Geometry check sheet. Reference: the model listing, model coordinates, mm. Face numbers are marked on the shaded views. A direction names the side the tool comes from. Coordinates: 2 decimals unless noted, no trailing zeros. Write each loop counter-clockwise with the first axis right and the second up, starting at its lowest first coordinate (ties: lowest second). Pieces come first, ordered by that corner, then holes. Notation, with made-up numbers: (73.25, 35.5) -> (110.25, 35.5) arc R28 cw to (110.25, 54.5) -> close; hole circle Ø3 at (-40, 82.25). An arc over 180 degrees is marked (long way). Put each result on its own line as item: value. Start each with the question number.
from build123d import *

# Parameters (mm, degrees)
SKETCH1_W           = 25
SKETCH1_H           = 52
BOSS_EXTRUDE1_DEPTH = 2
SKETCH2_W           = 25
SKETCH2_H           = 25
BOSS_EXTRUDE2_DEPTH = 2
SKETCH3_W           = 25
SKETCH3_H           = 25
BOSS_EXTRUDE3_DEPTH = 2
SKETCH5_R           = 4
CUT_EXTRUDE2_DEPTH  = 21
SKETCH6_R           = 1.5
CUT_EXTRUDE3_DEPTH  = 21
SKETCH7_R           = 2.5
CUT_EXTRUDE4_DEPTH  = 81


with BuildPart() as part:
    # Sketch1 → Boss-Extrude1 (new body)
    with BuildSketch(Plane.XY):
        with Locations((-0.174770451, 4.502942624)):
            Rectangle(SKETCH1_W, SKETCH1_H)
    extrude(amount=BOSS_EXTRUDE1_DEPTH)

    # Sketch2 → Boss-Extrude2 (add)
    with BuildSketch(Plane(origin=(0, 30.502942624, 0), x_dir=(1, 0, 0), z_dir=(0, 1, 0))):
        with Locations((-0.174770451, -12.5)):
            Rectangle(SKETCH2_W, SKETCH2_H)
    extrude(amount=BOSS_EXTRUDE2_DEPTH)

    # Sketch3 → Boss-Extrude3 (add)
    with BuildSketch(Plane(origin=(0, -21.497057376, 0), x_dir=(-1, 0, 0), z_dir=(0, -1, 0))):
        with Locations((0.174770451, -12.5)):
            Rectangle(SKETCH3_W, SKETCH3_H)
    extrude(amount=BOSS_EXTRUDE3_DEPTH)

    # Sketch5 → Cut-Extrude2 (cut)
    with BuildSketch(Plane(origin=(0, 0, 0), x_dir=(-1, 0, 0), z_dir=(0, 0, -1))):
        with Locations((0.174770451, 4.502942624)):
            Circle(SKETCH5_R)
    extrude(amount=-CUT_EXTRUDE2_DEPTH, mode=Mode.SUBTRACT)

    # Sketch6 → Cut-Extrude3 (cut)
    with BuildSketch(Plane(origin=(0, 0, 0), x_dir=(-1, 0, 0), z_dir=(0, 0, -1))):
        with Locations((7.174770451, 4.502942624)):
            Circle(SKETCH6_R)
        with Locations((0.174770451, -2.497057376)):
            Circle(SKETCH6_R)
        with Locations((-6.825229549, 4.502942624)):
            Circle(SKETCH6_R)
        with Locations((0.174770451, 11.502942624)):
            Circle(SKETCH6_R)
    extrude(amount=-CUT_EXTRUDE3_DEPTH, mode=Mode.SUBTRACT)

    # Sketch7 → Cut-Extrude4 (cut)
    with BuildSketch(Plane(origin=(0, -23.497057376, 0), x_dir=(-1, 0, 0), z_dir=(0, -1, 0))):
        with Locations(Location((0.174770451, -20, 0), (0, 0, 90))):
            Circle(SKETCH7_R)
    extrude(amount=-CUT_EXTRUDE4_DEPTH, mode=Mode.SUBTRACT)


solid = part.part
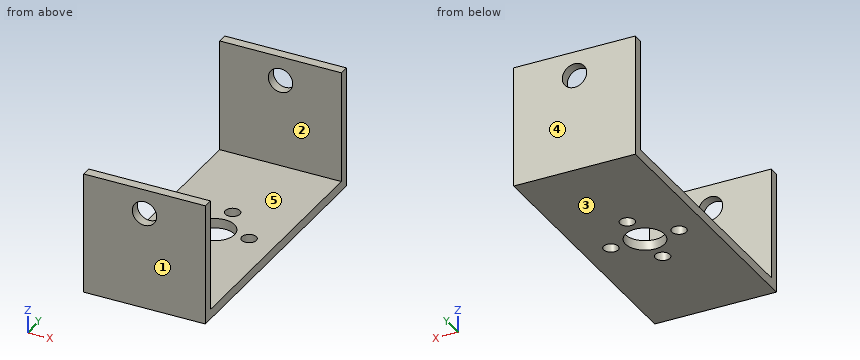
Item 1: Section check A-A, the plane z = 8.75. Enter the section's corners in (x, y), and give its area (3 significant figures).
Item 2: Access from +Z, -Z, +X, -X, +Y, -Y to the whole of each face (thin tool, end or side, straight path). Record for the marked faces 4 and 5.
Item 3: Go/stop test with a flat-tipped pin: P1, Ø5, axis at x = -0.17, y = 11.5, coming from the +Z side. Record where the tip stops, or that it passes through.
Item 4: Mould release check, pull along Y, two halves, no side actions. Record for the marked faces 1, 2 and 3: released by +Y, released by -Y, zero draft, split by the parting line, or undercut.
Item 5: Section check D-D, the plane x = 3.25. Enter the section's corners in (y, z), and give its area (3 significant figures).
Item 6: Scan lines: line 1 along Y through (x, z) = (-3, 17.75); line 2 along X through (y, z) = (-23, 20); line 3 along Z through (x, y) = (7.5, 27). Record each from-to range of solid material in increasing order. Write a range as [from, to].
Item 7: Section check C-C, the plane z = 20. Enter the section's corners in (x, y).
Item 8: Section check B-B, the plane x = 10.75. Enter the section's corners in (y, z), and give its area (3 significant figures).
From the geometry:
1. outline: (-12.67, -23.5) -> (12.33, -23.5) -> (12.33, -21.5) -> (-12.67, -21.5) -> close; (-12.67, 30.5) -> (12.33, 30.5) -> (12.33, 32.5) -> (-12.67, 32.5) -> close
1. area: 100 mm²
2. face 4: +Z, -Z, +X, -X, +Y
2. face 5: +Z, +X, -X
3. P1: z = 2
4. face 1: released by -Y
4. face 2: undercut
4. face 3: zero draft
5. outline: (-23.5, 0) -> (2.44, 0) -> (2.44, 2) -> (-21.5, 2) -> (-21.5, 25) -> (-23.5, 25) -> close; (6.57, 0) -> (32.5, 0) -> (32.5, 25) -> (30.5, 25) -> (30.5, 2) -> (6.57, 2) -> close
5. area: 196 mm²
6. line 1: [-23.5, -21.5], [30.5, 32.5]
6. line 2: [-12.67, -2.67], [2.33, 12.33]
6. line 3: [0, 2]
7. outline: (-12.67, -23.5) -> (-2.67, -23.5) -> (-2.67, -21.5) -> (-12.67, -21.5) -> close; (-12.67, 30.5) -> (-2.67, 30.5) -> (-2.67, 32.5) -> (-12.67, 32.5) -> close; (2.33, -23.5) -> (12.33, -23.5) -> (12.33, -21.5) -> (2.33, -21.5) -> close; (2.33, 30.5) -> (12.33, 30.5) -> (12.33, 32.5) -> (2.33, 32.5) -> close
8. outline: (-23.5, 0) -> (32.5, 0) -> (32.5, 25) -> (30.5, 25) -> (30.5, 2) -> (-21.5, 2) -> (-21.5, 25) -> (-23.5, 25) -> close
8. area: 204 mm²
